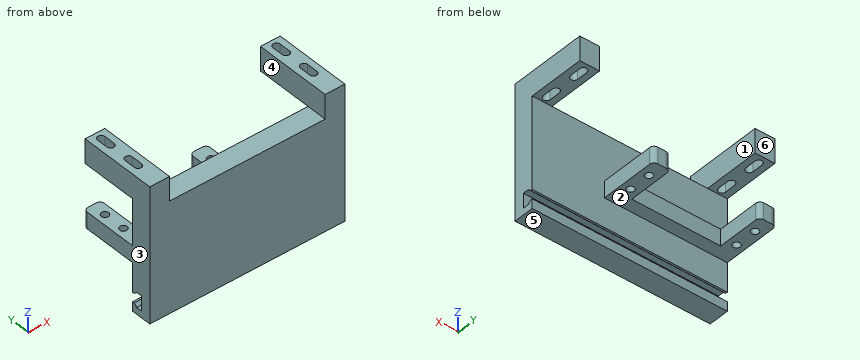
from build123d import *

# Parameters (mm, degrees)
SKETCH1_W           = 88.9
SKETCH1_H           = 39.25
BOSS_EXTRUDE1_DEPTH = 9.25
SKETCH2_W           = 56
SKETCH2_H           = 7.5
BOSS_EXTRUDE2_DEPTH = 26.49
SKETCH3_W           = 40.51
SKETCH3_H           = 20.88
CUT_EXTRUDE2_DEPTH  = 8.49
SKETCH5_R           = 1.675
CUT_EXTRUDE3_DEPTH  = 8.49
CUT_EXTRUDE4_DEPTH  = 91.49
FILLET1_R           = 2
FILLET2_R           = 2
SKETCH12_W          = 88.9
SKETCH12_H          = 9.25
BOSS_EXTRUDE3_DEPTH = 11
SKETCH16_W          = 9
SKETCH16_H          = 11
BOSS_EXTRUDE5_DEPTH = 35
CUT_EXTRUDE5_DEPTH  = 16
CUT_EXTRUDE6_DEPTH  = 16


with BuildPart() as part:
    # Sketch1 → Boss-Extrude1 (new body)
    with BuildSketch(Plane(origin=(0, 0, 0), x_dir=(1, 0, 0), z_dir=(0, 1, 0))):
        Rectangle(SKETCH1_W, SKETCH1_H)
    extrude(amount=BOSS_EXTRUDE1_DEPTH)

    # Sketch2 → Boss-Extrude2 (add)
    with BuildSketch(Plane(origin=(0, 9.25, 0), x_dir=(1, 0, 0), z_dir=(0, 1, 0))):
        with Locations((-16.45, -5.848195432)):
            Rectangle(SKETCH2_W, SKETCH2_H)
    extrude(amount=BOSS_EXTRUDE2_DEPTH)

    # Sketch3 → Cut-Extrude2 (cut)
    with BuildSketch(Plane.XY.offset(9.598195432)):
        with Locations((-16.45, 25.3)):
            Rectangle(SKETCH3_W, SKETCH3_H)
    extrude(amount=-CUT_EXTRUDE2_DEPTH, mode=Mode.SUBTRACT)

    # Sketch5 → Cut-Extrude3 (cut)
    with BuildSketch(Plane.XY.offset(9.598195432)):
        with Locations((-40.6, 18.82)):
            Circle(SKETCH5_R)
        with Locations((-40.6, 28.82)):
            Circle(SKETCH5_R)
        with Locations((7.7, 18.82)):
            Circle(SKETCH5_R)
        with Locations((7.7, 28.82)):
            Circle(SKETCH5_R)
    extrude(amount=-CUT_EXTRUDE3_DEPTH, mode=Mode.SUBTRACT)

    # Sketch10 → Cut-Extrude4 (cut)
    with BuildSketch(Plane.ZY.offset(44.45)):
        Polygon((-16.575, 4.44331134), (-9.845, 4.44331134), (-9.845, 7.11331134), (-11.117792206, 8.386103546), (-11.115, 9.25), (-15.305, 9.25), (-15.302207794, 8.386103546), (-16.575, 7.11331134), align=None)
    extrude(amount=-CUT_EXTRUDE4_DEPTH, mode=Mode.SUBTRACT)

    # Fillet1
    fillet1_edges = [part.edges().sort_by_distance(p)[0] for p in [
        (-44.45, 35.74, 5.848195432),
        (-36.705, 35.74, 5.848195432),
    ]]
    fillet(fillet1_edges, radius=FILLET1_R)

    # Fillet2
    fillet2_edges = [part.edges().sort_by_distance(p)[0] for p in [
        (11.55, 35.74, 5.848195432),
        (3.805, 35.74, 5.848195432),
    ]]
    fillet(fillet2_edges, radius=FILLET2_R)

    # Sketch12 → Boss-Extrude3 (add)
    with BuildSketch(Plane.XY.offset(19.625)):
        with Locations((0, 4.625)):
            Rectangle(SKETCH12_W, SKETCH12_H)
    extrude(amount=BOSS_EXTRUDE3_DEPTH)

    # Sketch16 → Boss-Extrude5 (add)
    with BuildSketch(Plane(origin=(0, 0, 0), x_dir=(1, 0, 0), z_dir=(0, 1, 0))):
        with Locations((39.95, -36.125)):
            Rectangle(SKETCH16_W, SKETCH16_H)
    boss_extrude5 = extrude(amount=BOSS_EXTRUDE5_DEPTH)

    # Sketch17 → Cut-Extrude5 (cut)
    with BuildSketch(Plane(origin=(0, 0, 30.625), x_dir=(-1, 0, 0), z_dir=(0, 0, -1))):
        with BuildLine():
            Line((-41.575, 11.71), (-41.575, 16.79))
            ThreePointArc((-41.575, 16.79), (-39.95, 18.415), (-38.325, 16.79))
            Line((-38.325, 16.79), (-38.325, 11.71))
            ThreePointArc((-38.325, 11.71), (-39.95, 10.085), (-41.575, 11.71))
        make_face()
    cut_extrude5 = extrude(amount=-CUT_EXTRUDE5_DEPTH, mode=Mode.SUBTRACT)

    # Sketch19 → Cut-Extrude6 (cut)
    with BuildSketch(Plane(origin=(0, 0, 30.625), x_dir=(-1, 0, 0), z_dir=(0, 0, -1))):
        with BuildLine():
            Line((-41.575, 26.546678497), (-41.575, 31.626678497))
            ThreePointArc((-41.575, 31.626678497), (-39.95, 33.251678497), (-38.325, 31.626678497))
            Line((-38.325, 31.626678497), (-38.325, 26.546678497))
            ThreePointArc((-38.325, 26.546678497), (-39.95, 24.921678497), (-41.575, 26.546678497))
        make_face()
    cut_extrude6 = extrude(amount=-CUT_EXTRUDE6_DEPTH, mode=Mode.SUBTRACT)

    # Mirror1: Boss-Extrude5, Cut-Extrude5, Cut-Extrude6 across plane
    add(boss_extrude5.mirror(Plane(origin=(0, 0, 0), x_dir=(0, 0, 1), z_dir=(1, 0, 0))))
    add(cut_extrude5.mirror(Plane(origin=(0, 0, 0), x_dir=(0, 0, 1), z_dir=(1, 0, 0))), mode=Mode.SUBTRACT)
    add(cut_extrude6.mirror(Plane(origin=(0, 0, 0), x_dir=(0, 0, 1), z_dir=(1, 0, 0))), mode=Mode.SUBTRACT)


solid = part.part
Input: part model. Units: mm. Frame: model coordinates. Face numbers are marked on the shaded views. A direction names the side the tool comes from. Coordinates: 2 decimals unless noted, no trailing zeros. Order: outer loops, then holes, each group sorted by start corner. A loop starts at its lowest first (then second) coordinate and runs counter-clockwise, first axis right, second up. Notation, with made-up numbers: M 83.25,-23 L 115.25,-23 A14 ccw 115.25,-17 Z; hole C 17.5,51.25 d1. An arc over 180 degrees is marked long. Answer in a Markdown table with one row per item.
(1) Draft query along X for the marked faces 1, 2 and 3. Return one class per face: pulls with the +X half, pulls with the -X half, needs draft (parallel to the pull), parting line crosses it, or undercut.
Numbers:
| item | result |
|---|---|
| face 1 | undercut |
| face 2 | needs draft |
| face 3 | pulls with the -X half |
(2) Section query A-A, the plane y = 21.5. Output: boundary loops of the cut face in (x, z) (3 decimals).
Numbers:
| item | result |
|---|---|
| outline | M -44.45,2.098 L -36.705,2.098 L -36.705,9.598 L -44.45,9.598 Z; M -44.45,30.625 L -35.45,30.625 L -35.45,41.625 L -44.45,41.625 Z; M 3.805,2.098 L 11.55,2.098 L 11.55,9.598 L 3.805,9.598 Z; M 35.45,30.625 L 44.45,30.625 L 44.45,41.625 L 35.45,41.625 Z |
(3) Section query D-D, the plane x = -33. Output: boundary loops of the cut face in (y, z) (3 decimals), plus the area to 3 significant figures.
Numbers:
| item | result |
|---|---|
| outline | M 0,-19.625 L 9.25,-19.625 L 9.25,-15.305 L 8.386,-15.302 L 7.113,-16.575 L 4.443,-16.575 L 4.443,-9.845 L 7.113,-9.845 L 8.386,-11.118 L 9.25,-11.115 L 9.25,2.098 L 14.86,2.098 L 14.86,9.598 L 9.25,9.598 L 9.25,30.625 L 0,30.625 Z |
| area | 478 mm^2 |
(4) Section query C-C, the plane y = 28.82. Give the number of separate pieces and of enclosed holes in the cut face, plus the area to 3 significant figures.
Numbers:
| item | result |
|---|---|
| separate pieces | 8 |
| enclosed holes | 0 |
| area | 192 mm^2 |
(5) Material intervals for line 1 (Y direction, x = 7.7, z = 5.5) (3 decimals); line 2 (X direction, y = 30, z = 35) (3 decimals); line 3 (X direction, y = 26.5, z = 6.5) (3 decimals), sorted ascending. Write a range as [from, to].
Numbers:
| item | result |
|---|---|
| line 1 | y = [0, 17.145], [20.495, 27.145], [30.495, 35.74] |
| line 2 | x = [-44.45, -41.575], [-38.325, -35.45], [35.45, 38.325], [41.575, 44.45] |
| line 3 | x = [-44.45, -36.705], [3.805, 11.55] |
(6) Contact query for flat-ended pins moving along their axis: pin 1 Ø10 at (x, z) = (-19, 16.5) entering from +Y; pin 2 Ø4 at (y, z) = (26.5, 6) entering from +X; pin 3 Ø4 at (x, z) = (-22.5, 5) entering from +Y; pin 4 Ø10 at (y, z) = (31, 19.5) entering from +X. Output: stop coordinate, or through.
Numbers:
| item | result |
|---|---|
| pin 1 | stops at y = 9.25 |
| pin 2 | stops at x = 11.55 |
| pin 3 | stops at y = 14.86 |
| pin 4 | passes through |
(7) Section query B-B, the plane x = 7.7. Output: boundary loops of the cut face in (y, z) (3 decimals), plus the area to 3 significant figures.
Numbers:
| item | result |
|---|---|
| outline | M 0,-19.625 L 9.25,-19.625 L 9.25,-15.305 L 8.386,-15.302 L 7.113,-16.575 L 4.443,-16.575 L 4.443,-9.845 L 7.113,-9.845 L 8.386,-11.118 L 9.25,-11.115 L 9.25,2.098 L 17.145,2.098 L 17.145,9.598 L 9.25,9.598 L 9.25,30.625 L 0,30.625 Z; M 20.495,2.098 L 27.145,2.098 L 27.145,9.598 L 20.495,9.598 Z; M 30.495,2.098 L 35.74,2.098 L 35.74,9.598 L 30.495,9.598 Z |
| area | 585 mm^2 |
(8) Access query for the marked faces 4, 5 and 6. Directions: +Z, -Z, +X, -X, +Y, -Y. A direction counts if a zero-diameter tool reaches every point of the face in a straight line with its end or side. Return the directions, or none.
Numbers:
| item | result |
|---|---|
| face 4 | +Z, +Y, -Y |
| face 5 | -Z, +X, -X, +Y, -Y |
| face 6 | +Z, +X, -X, +Y |
